from build123d import *

# Parameters (mm, degrees)
ESBO_O1_R             = 5.35
FLANGE_BASE1_DEPTH    = 5
CORTE_EXTRUS_O1_REACH = 58.115
ESBO_O2_R             = 1
QUEBRA_CANTO1_START   = -5
QUEBRA_CANTO1_DEPTH   = 5


# Read off the part's stored shape, not the designer's step: Quebra-Canto1
# Sheet-metal steps are written as plain solids
with BuildPart() as part:
    # Esboço1 → Flange-base1 (new body)
    with BuildSketch(Plane.XY):
        Polygon((19.699698823, 8.736399513), (12.699698794, 8.736399513), (12.699698794, -1.263600636), (19.699698823, -1.263600636), (19.699698823, -20.26360068), (24.199698913, -20.26360068), (24.199698913, -25.263600799), (19.699698982, -25.263600562), (19.699698823, -28.263600308), (19.699698823, -33.263600919), (-30.300301832, -33.263600919), (-30.300301832, -28.263600308), (-30.30030199, -25.263600562), (-34.800301922, -25.263600799), (-34.800301922, -20.26360068), (-30.300301832, -20.26360068), (-30.300301832, -1.263600636), (-23.300301802, -1.263600636), (-23.300301802, 8.736399513), (-30.300301832, 8.736399513), (-30.300301832, 17.736399558), (-34.800301922, 17.736399558), (-34.800301922, 27.736399558), (-30.300301832, 27.736399558), (-30.300301832, 31.736399692), (-23.500301773, 31.736399692), (-23.500301773, 30.536399744), (-21.100301772, 30.536399744), (-21.100301772, 31.736399692), (-19.300301772, 31.736399692), (-19.300301772, 34.736399796), (-21.100301772, 34.736399796), (-21.100301772, 35.936399744), (-23.500301772, 35.936399744), (-23.500301772, 34.736399796), (-30.300301832, 34.736399796), (-30.300301832, 38.736399796), (-34.800301832, 38.736399796), (-34.800301832, 43.736399796), (24.199698817, 43.736399796), (24.199698817, 38.736399797), (19.699698817, 38.736399797), (19.699698817, 34.736399797), (12.899698227, 34.736399797), (12.899698227, 35.936399744), (10.499698227, 35.936399744), (10.499698227, 34.736399797), (8.699698168, 34.736399797), (8.699698168, 31.736399692), (10.499698227, 31.736399692), (10.499698227, 30.536399751), (12.899698233, 30.536399751), (12.899698233, 31.736399692), (19.699698823, 31.736399692), (19.699698823, 27.736399558), (24.199698913, 27.736399558), (24.199698913, 17.736399558), (19.699698823, 17.736399558), align=None)
        with Locations((-5.300301504, 3.736399439)):
            Circle(ESBO_O1_R, mode=Mode.SUBTRACT)
    extrude(amount=-FLANGE_BASE1_DEPTH)

    # Esboço2 → Corte-extrusão1 (cut, up to next)
    with BuildSketch(Plane.XY, mode=Mode.PRIVATE) as corte_extrus_o1_sk1:
        with Locations((-30.300301832, 38.736399796)):
            Circle(ESBO_O2_R)
    corte_extrus_o1_tool1 = extrude(corte_extrus_o1_sk1.sketch, amount=-CORTE_EXTRUS_O1_REACH, mode=Mode.PRIVATE) & part.part
    # Esboço2 → Corte-extrusão1 (cut, up to next)
    with BuildSketch(Plane.XY, mode=Mode.PRIVATE) as corte_extrus_o1_sk2:
        with Locations((-30.300301832, 27.736399558)):
            Circle(ESBO_O2_R)
    corte_extrus_o1_tool2 = extrude(corte_extrus_o1_sk2.sketch, amount=-CORTE_EXTRUS_O1_REACH, mode=Mode.PRIVATE) & part.part
    # Esboço2 → Corte-extrusão1 (cut, up to next)
    with BuildSketch(Plane.XY, mode=Mode.PRIVATE) as corte_extrus_o1_sk3:
        with Locations((-30.300301832, 17.736399558)):
            Circle(ESBO_O2_R)
    corte_extrus_o1_tool3 = extrude(corte_extrus_o1_sk3.sketch, amount=-CORTE_EXTRUS_O1_REACH, mode=Mode.PRIVATE) & part.part
    # Esboço2 → Corte-extrusão1 (cut, up to next)
    with BuildSketch(Plane.XY, mode=Mode.PRIVATE) as corte_extrus_o1_sk4:
        with Locations((-23.300301802, 8.736399513)):
            Circle(ESBO_O2_R)
    corte_extrus_o1_tool4 = extrude(corte_extrus_o1_sk4.sketch, amount=-CORTE_EXTRUS_O1_REACH, mode=Mode.PRIVATE) & part.part
    # Esboço2 → Corte-extrusão1 (cut, up to next)
    with BuildSketch(Plane.XY, mode=Mode.PRIVATE) as corte_extrus_o1_sk5:
        with Locations((-23.300301802, -1.263600636)):
            Circle(ESBO_O2_R)
    corte_extrus_o1_tool5 = extrude(corte_extrus_o1_sk5.sketch, amount=-CORTE_EXTRUS_O1_REACH, mode=Mode.PRIVATE) & part.part
    # Esboço2 → Corte-extrusão1 (cut, up to next)
    with BuildSketch(Plane.XY, mode=Mode.PRIVATE) as corte_extrus_o1_sk6:
        with Locations((-30.300301832, -20.26360068)):
            Circle(ESBO_O2_R)
    corte_extrus_o1_tool6 = extrude(corte_extrus_o1_sk6.sketch, amount=-CORTE_EXTRUS_O1_REACH, mode=Mode.PRIVATE) & part.part
    # Esboço2 → Corte-extrusão1 (cut, up to next)
    with BuildSketch(Plane.XY, mode=Mode.PRIVATE) as corte_extrus_o1_sk7:
        with Locations((-30.30030199, -25.263600562)):
            Circle(ESBO_O2_R)
    corte_extrus_o1_tool7 = extrude(corte_extrus_o1_sk7.sketch, amount=-CORTE_EXTRUS_O1_REACH, mode=Mode.PRIVATE) & part.part
    # Esboço2 → Corte-extrusão1 (cut, up to next)
    with BuildSketch(Plane.XY, mode=Mode.PRIVATE) as corte_extrus_o1_sk8:
        with Locations((19.699698982, -25.263600562)):
            Circle(ESBO_O2_R)
    corte_extrus_o1_tool8 = extrude(corte_extrus_o1_sk8.sketch, amount=-CORTE_EXTRUS_O1_REACH, mode=Mode.PRIVATE) & part.part
    # Esboço2 → Corte-extrusão1 (cut, up to next)
    with BuildSketch(Plane.XY, mode=Mode.PRIVATE) as corte_extrus_o1_sk9:
        with Locations((19.699698823, -20.26360068)):
            Circle(ESBO_O2_R)
    corte_extrus_o1_tool9 = extrude(corte_extrus_o1_sk9.sketch, amount=-CORTE_EXTRUS_O1_REACH, mode=Mode.PRIVATE) & part.part
    # Esboço2 → Corte-extrusão1 (cut, up to next)
    with BuildSketch(Plane.XY, mode=Mode.PRIVATE) as corte_extrus_o1_sk10:
        with Locations((12.699698794, 8.736399513)):
            Circle(ESBO_O2_R)
    corte_extrus_o1_tool10 = extrude(corte_extrus_o1_sk10.sketch, amount=-CORTE_EXTRUS_O1_REACH, mode=Mode.PRIVATE) & part.part
    # Esboço2 → Corte-extrusão1 (cut, up to next)
    with BuildSketch(Plane.XY, mode=Mode.PRIVATE) as corte_extrus_o1_sk11:
        with Locations((12.699698794, -1.263600636)):
            Circle(ESBO_O2_R)
    corte_extrus_o1_tool11 = extrude(corte_extrus_o1_sk11.sketch, amount=-CORTE_EXTRUS_O1_REACH, mode=Mode.PRIVATE) & part.part
    # Esboço2 → Corte-extrusão1 (cut, up to next)
    with BuildSketch(Plane.XY, mode=Mode.PRIVATE) as corte_extrus_o1_sk12:
        with Locations((19.699698823, 17.736399558)):
            Circle(ESBO_O2_R)
    corte_extrus_o1_tool12 = extrude(corte_extrus_o1_sk12.sketch, amount=-CORTE_EXTRUS_O1_REACH, mode=Mode.PRIVATE) & part.part
    # Esboço2 → Corte-extrusão1 (cut, up to next)
    with BuildSketch(Plane.XY, mode=Mode.PRIVATE) as corte_extrus_o1_sk13:
        with Locations((19.699698817, 38.736399797)):
            Circle(ESBO_O2_R)
    corte_extrus_o1_tool13 = extrude(corte_extrus_o1_sk13.sketch, amount=-CORTE_EXTRUS_O1_REACH, mode=Mode.PRIVATE) & part.part
    # Esboço2 → Corte-extrusão1 (cut, up to next)
    with BuildSketch(Plane.XY, mode=Mode.PRIVATE) as corte_extrus_o1_sk14:
        with Locations((19.699698823, 27.736399558)):
            Circle(ESBO_O2_R)
    corte_extrus_o1_tool14 = extrude(corte_extrus_o1_sk14.sketch, amount=-CORTE_EXTRUS_O1_REACH, mode=Mode.PRIVATE) & part.part
    add(corte_extrus_o1_tool1.solids().sort_by_distance((-30.300302, 38.7364, 0))[0], mode=Mode.SUBTRACT)
    add(corte_extrus_o1_tool2.solids().sort_by_distance((-30.300302, 27.7364, 0))[0], mode=Mode.SUBTRACT)
    add(corte_extrus_o1_tool3.solids().sort_by_distance((-30.300302, 17.7364, 0))[0], mode=Mode.SUBTRACT)
    add(corte_extrus_o1_tool4.solids().sort_by_distance((-23.300302, 8.7364, 0))[0], mode=Mode.SUBTRACT)
    add(corte_extrus_o1_tool5.solids().sort_by_distance((-23.300302, -1.263601, 0))[0], mode=Mode.SUBTRACT)
    add(corte_extrus_o1_tool6.solids().sort_by_distance((-30.300302, -20.263601, 0))[0], mode=Mode.SUBTRACT)
    add(corte_extrus_o1_tool7.solids().sort_by_distance((-30.300302, -25.263601, 0))[0], mode=Mode.SUBTRACT)
    add(corte_extrus_o1_tool8.solids().sort_by_distance((19.699699, -25.263601, 0))[0], mode=Mode.SUBTRACT)
    add(corte_extrus_o1_tool9.solids().sort_by_distance((19.699699, -20.263601, 0))[0], mode=Mode.SUBTRACT)
    add(corte_extrus_o1_tool10.solids().sort_by_distance((12.699699, 8.7364, 0))[0], mode=Mode.SUBTRACT)
    add(corte_extrus_o1_tool11.solids().sort_by_distance((12.699699, -1.263601, 0))[0], mode=Mode.SUBTRACT)
    add(corte_extrus_o1_tool12.solids().sort_by_distance((19.699699, 17.7364, 0))[0], mode=Mode.SUBTRACT)
    add(corte_extrus_o1_tool13.solids().sort_by_distance((19.699699, 38.7364, 0))[0], mode=Mode.SUBTRACT)
    add(corte_extrus_o1_tool14.solids().sort_by_distance((19.699699, 27.7364, 0))[0], mode=Mode.SUBTRACT)

    # Quebra-Canto1 outline → Quebra-Canto1 (add)
    with BuildSketch(Plane.XY.offset(QUEBRA_CANTO1_START)):
        with BuildLine():
            Line((8.699698168, 34.736399797), (8.699698168, 34.236399797))
            ThreePointArc((8.699698168, 34.236399797), (8.846144777, 34.589953188), (9.199698168, 34.736399797))
            Line((9.199698168, 34.736399797), (8.699698168, 34.736399797))
        make_face()
        with BuildLine():
            ThreePointArc((9.199698168, 31.736399692), (8.846144777, 31.882846301), (8.699698168, 32.236399692))
            Line((8.699698168, 32.236399692), (8.699698168, 31.736399692))
            Line((8.699698168, 31.736399692), (9.199698168, 31.736399692))
        make_face()
        with BuildLine():
            Line((-19.300301772, 31.736399692), (-19.300301772, 32.236399692))
            ThreePointArc((-19.300301772, 32.236399692), (-19.446748382, 31.882846301), (-19.800301772, 31.736399692))
            Line((-19.800301772, 31.736399692), (-19.300301772, 31.736399692))
        make_face()
        with BuildLine():
            ThreePointArc((-19.800301772, 34.736399796), (-19.446748382, 34.589953186), (-19.300301772, 34.236399796))
            Line((-19.300301772, 34.236399796), (-19.300301772, 34.736399796))
            Line((-19.300301772, 34.736399796), (-19.800301772, 34.736399796))
        make_face()
    extrude(amount=QUEBRA_CANTO1_DEPTH)


solid = part.part
Work out the finished part from the listing and answer in its coordinate system (mm). A direction names the side the tool comes from. Give positions to 0.01 mm unless a question says otherwise; leave off trailing zeros. Order: outer loops, then holes, each group sorted by start corner. A loop starts at its lowest first (then second) coordinate and runs counter-clockwise, first axis right, second up. Notation, with made-up numbers: (67, 70.5) -> (114, 70.5) arc R28 cw to (114, 103.5) -> close; hole circle Ø11 at (8.5, 4.5). An arc over 180 degrees is marked (long way). Answer as a JSON object with one key per item and string values. Group by question number.
1. Section B-B on y = 1 is taken. Determine the outline of the cut face in (x, z).
2. A tool of negligible diameter and unlimited length cuts with its end or side. For faces 4 (the flat face through (-12, 6, 0)), 5 (the flat face through (-22, 30.536, -2)), 6 (the flat face through (22, 17.736, -2)), 7 (the flat face through (-27, 31.736, -2)), 8 (the flat face through (22, -25.264, -2)), from which of +Z, -Z, +X, -X, +Y, -Y can it reach the whole face along a straight path? Write none if from no direction.
3. Flat-ended cylindrical pins translate along their axes: pin 1 Ø2.5 at (y, z) = (-11, -3) entering from -X; pin 2 Ø1.5 at (x, y) = (-20, 19.5) entering from +Z; pin 3 Ø1.5 at (y, z) = (4, -3.5) entering from +X; pin 4 Ø0.6 at (y, z) = (31.5, -3.5) entering from +X. Find the tip coordinate at first contact, or state that the pin passes through.
4. Section A-A on x = -7.5 is taken. Determine the outline of the cut face in (y, z), plus the area to 3 significant figures.
5. Consider line 1 along Y through (x, z) = (-29, -3.5); line 2 along Y through (x, z) = (11.5, -3.8); line 3 along Y through (x, z) = (-23, -1.75). Determine where each line is inside the solid, lowest interval first. Write a range as [from, to].
6. The mould has two halves that part along Y. Classify faces 1 (the flat face through (24.2, 41, -2)), 2 (the flat face through (-33, -25.264, -2)), 3 (the flat face through (22, 38.736, -2)): released by +Y, released by -Y, zero draft, split by the parting line, or undercut.
7. Section C-C on y = 15 is taken. Determine the outline of the cut face in (x, z).
Result sheet:
{
 "1": {"outline": "(-23.3, -5) -> (-9.9, -5) -> (-9.9, 0) -> (-23.3, 0) -> close; (-0.7, -5) -> (12.7, -5) -> (12.7, 0) -> (-0.7, 0) -> close"},
 "2": {"face 4": "+Z, +X, -X, +Y, -Y", "face 5": "+Z, -Z", "face 6": "+Z, -Z, +X", "face 7": "+Z, -Z, -X", "face 8": "+Z, -Z, +X, -Y"},
 "3": {"pin 1": "stops at x = -30.3", "pin 2": "stops at z = 0", "pin 3": "stops at x = 12.7", "pin 4": "stops at x = 19.7"},
 "4": {"outline": "(-33.26, -5) -> (-1.14, -5) -> (-1.14, 0) -> (-33.26, 0) -> close; (8.61, -5) -> (43.74, -5) -> (43.74, 0) -> (8.61, 0) -> close", "area": "336 mm^2"},
 "5": {"line 1": "y = [-33.26, -1.26], [8.74, 31.74], [34.74, 43.74]", "line 2": "y = [-33.26, 30.54], [35.94, 43.74]", "line 3": "y = [-33.26, -2.22], [-0.31, 7.78], [9.69, 30.54], [35.94, 43.74]"},
 "6": {"face 1": "zero draft", "face 2": "released by -Y", "face 3": "undercut"},
 "7": {"outline": "(-30.3, -5) -> (19.7, -5) -> (19.7, 0) -> (-30.3, 0) -> close"}
}
